from build123d import *

# Parameters (mm, degrees)
SKETCH1_W           = 210
SKETCH1_H           = 200
BOSS_EXTRUDE1_DEPTH = 30
SKETCH2_W           = 194
SKETCH2_H           = 20
CUT_EXTRUDE1_DEPTH  = 228.870577302
CUT_EXTRUDE2_DEPTH  = 149.07092895
CUT_EXTRUDE3_DEPTH  = 149.07092895
SKETCH6_W           = 183.698961066
SKETCH6_H           = 20
CUT_EXTRUDE4_DEPTH  = 147.372811683
CUT_EXTRUDE6_DEPTH  = 5


with BuildPart() as part:
    # Sketch1 → Boss-Extrude1 (new body)
    with BuildSketch(Plane.XY):
        Rectangle(SKETCH1_W, SKETCH1_H)
    extrude(amount=BOSS_EXTRUDE1_DEPTH)

    # Sketch2 → Cut-Extrude1 (cut, through all)
    with BuildSketch(Plane(origin=(0, -100, 0), x_dir=(-1, 0, 0), z_dir=(0, -1, 0))):
        with Locations((0, -10)):
            Rectangle(SKETCH2_W, SKETCH2_H)
    extrude(amount=-CUT_EXTRUDE1_DEPTH, mode=Mode.SUBTRACT)

    # Sketch3 → Cut-Extrude2 (cut, through all)
    with BuildSketch(Plane.XY.offset(30)):
        with BuildLine():
            Line((88, 85), (88, -45))
            ThreePointArc((88, -45), (91.5, -48.5), (95, -45))
            Line((95, -45), (95, 85))
            ThreePointArc((95, 85), (91.5, 88.5), (88, 85))
        make_face()
    extrude(amount=-CUT_EXTRUDE2_DEPTH, mode=Mode.SUBTRACT)

    # Sketch4 → Cut-Extrude3 (cut, through all)
    with BuildSketch(Plane.XY.offset(30)):
        with BuildLine():
            Line((91.5, 83), (-95, 83))
            ThreePointArc((-95, 83), (-98.5, 86.5), (-95, 90))
            Line((-95, 90), (91.5, 90))
            ThreePointArc((91.5, 90), (95, 86.5), (91.5, 83))
        make_face()
    extrude(amount=-CUT_EXTRUDE3_DEPTH, mode=Mode.SUBTRACT)

    # Sketch6 → Cut-Extrude4 (cut, through all)
    with BuildSketch(Plane(origin=(0, 0, 20), x_dir=(-1, 0, 0), z_dir=(0, 0, -1))):
        with Locations((-1.082669049, -62.138985898)):
            Rectangle(SKETCH6_W, SKETCH6_H)
    extrude(amount=-CUT_EXTRUDE4_DEPTH, mode=Mode.SUBTRACT)

    # Sketch5 → Cut-Extrude6 (cut)
    with BuildSketch(Plane(origin=(0, -100, 0), x_dir=(-1, 0, 0), z_dir=(0, -1, 0))):
        with BuildLine():
            Line((90, -27), (-90, -27))
            ThreePointArc((-90, -27), (-92.5, -24.5), (-90, -22))
            Line((-90, -22), (90, -22))
            ThreePointArc((90, -22), (92.5, -24.5), (90, -27))
        make_face()
    extrude(amount=-CUT_EXTRUDE6_DEPTH, mode=Mode.SUBTRACT)


solid = part.part
Build history of the part. All positions in model axes, mm. A direction names the side the tool comes from. Coordinates: 2 decimals unless noted, no trailing zeros. Order: outer loops, then holes, each group sorted by start corner. A loop starts at its lowest first (then second) coordinate and runs counter-clockwise, first axis right, second up. Notation, with made-up numbers: (44, 15.25) - (62, 15.25) arc R23 cw to (62, 29.25) - close; hole circle Ø5 at (2.25, 85.5). An arc over 180 degrees is marked (long way). Write item = value, one per line. Start each with the question number.
1) Saw through at A-A on z = 12.75. Write the cut outline in (x, y), then the cut area to 3 significant figures.
2) Saw through at B-B on y = 29. Write the cut outline in (x, z).
3) Wall check: line 1 along Y through (x, z) = (82, 21.5); line 2 along Y through (x, z) = (56, 23.25); line 3 along X through (y, z) = (69.5, 7.5). Give the ranges that are in metal, low to high. Write a range as from..to.
4) Saw through at D-D on z = 24.5. Write the cut outline in (x, y).
5) 3-axis set-ups, long thin cutter, end or side, ignore diameter. For faces 1 (the face through (2, -52.139, 25)), 2 (the face through (-101, 1, 0)), 3 (the face through (1, -1, 20)), 4 (the face through (1, -98, 22)): which of +Z, -Z, +X, -X, +Y, -Y reach the whole face in a straight line?
6) Flat gauge pins, fed straight in: pin 1 Ø8 at (x, z) = (-43.5, 24.5) entering from -Y; pin 2 Ø2.5 at (x, z) = (-41.5, 24) entering from -Y; pin 3 Ø3 at (x, y) = (-77, -21.5) entering from -Z. Where does each tip first touch, or does it go through?
7) Two-plate mould, pull along X, no slides. Class faces 5 (the face through (-1, 1, 30)), 6 (the face through (105, -1, 15)), 7 (the face through (-98.5, 86.4, 18.5)): pulls with the +X half, pulls with the -X half, needs draft (parallel to the pull), parting line crosses it, or undercut.
8) Saw through at C-C on x = 23. Write the cut outline in (y, z), then the cut area to 4 significant figures.
From the geometry:
q1.outline = (-105, -100) - (-97, -100) - (-97, 83.63) arc R3.5 cw to (-97, 89.37) - (-97, 100) - (-105, 100) - close; (97, -100) - (105, -100) - (105, 100) - (97, 100) - close
q1.area = 3,190 mm^2
q2.outline = (-105, 0) - (-97, 0) - (-97, 20) - (88, 20) - (88, 30) - (-105, 30) - close; (95, 20) - (97, 20) - (97, 0) - (105, 0) - (105, 30) - (95, 30) - close
q3.line_1 = -100..-72.14, -52.14..83, 90..100
q3.line_2 = -95..-72.14, -52.14..83, 90..100
q3.line_3 = -105..-97, 97..105
q4.outline = (-105, -100) - (-92.5, -100) - (-92.5, -95) - (92.5, -95) - (92.5, -100) - (105, -100) - (105, 100) - (-105, 100) - close; hole (-95, 83) - (88, 83) - (88, -45) arc R3.5 ccw to (95, -45) - (95, 85) arc R3.5 ccw to (94.92, 85.75) arc R3.5 ccw to (91.5, 90) - (-95, 90) arc R3.5 ccw to start; hole (-90.77, -72.14) - (92.93, -72.14) - (92.93, -52.14) - (-90.77, -52.14) - close
q5.face_1 = +Z, -Z
q5.face_2 = -Z, +X, -X, +Y, -Y
q5.face_3 = -Z, +Y, -Y
q5.face_4 = -Y
q6.pin_1 = -100
q6.pin_2 = -95
q6.pin_3 = 20
q7.face_5 = needs draft
q7.face_6 = pulls with the +X half
q7.face_7 = undercut
q8.outline = (-100, 20) - (-72.14, 20) - (-72.14, 30) - (-100, 30) - (-100, 27) - (-95, 27) - (-95, 22) - (-100, 22) - close; (-52.14, 20) - (83, 20) - (83, 30) - (-52.14, 30) - close; (90, 20) - (100, 20) - (100, 30) - (90, 30) - close
q8.area = 1,705 mm^2
